Autodesk Fusion 360 part; units mm, degrees
sketch "Outer" plane through (0, 0, 0) normal (0, 1, 0) x (1, 0, 0)
  circle A0 centre (0, 0) radius 12.5
  dimension "d1" = 25
extrude "Outer Extrusion" add sketch "Outer" along normal blind 20
sketch "Inner" plane through (0, 20, 0) normal (0, 1, 0) x (-1, 0, 0)
  circle A0 centre (0, 0) radius 12.5
  circle A1 centre (0, 0) radius 10.5
  dimension "d4" = 21
extrude "Inner Extrusion" cut sketch "Inner" against normal blind 18 contours A1
sketch "Shaft" plane through (0, 2, 0) normal (0, 1, 0) x (-1, 0, 0)
  circle A0 centre (0, 0) radius 10.5
  line L0 (-1.7, 2.5923) -> (-1.7, -2.5923)
  arc A1 (-1.7, -2.5923) -> (-1.7, 2.5923) centre (0, 0) ccw
  arc A2 (-3.7, -3.51) -> (-3.7, 3.51) centre (0, 0) ccw
  line L1 (-3.7, 3.51) -> (-3.7, -3.51)
  dimension "d7" = 6.2
  dimension "d8" = 1.7
  dimension "d9" = 2
extrude "Shaft Extrusion" add sketch "Shaft" along normal blind 12.5 contours A2 L1
equation "d4 = 25 mm - 2 mm - 2 mm"
equation "d5 = -( 20 mm - 2 mm )"
equation "d7 = 5.8 mm + 0.2 mm + 0.2 mm"
equation "d8 = ( 4.5 mm - 3 mm ) + 0.2 mm"
equation "d10 = 20 mm - 2 mm - 5.5 mm"
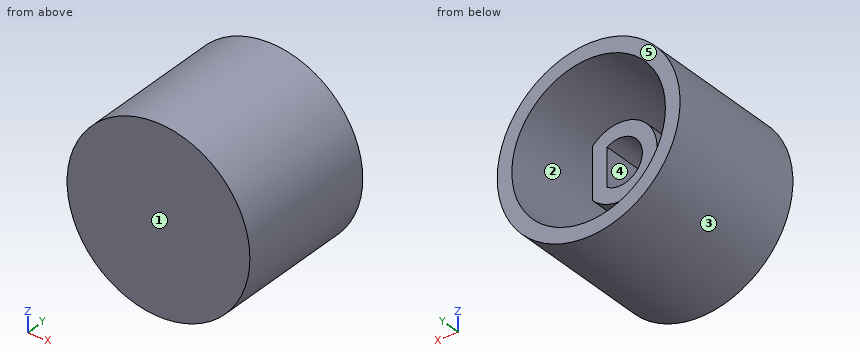
Check sheet for the modelled part. Datum: model origin and axes. Units: mm. Face numbers are marked on the shaded views. A direction names the side the tool comes from. Round coordinates to 2 decimals unless told otherwise and drop trailing zeros. Write each loop counter-clockwise with the first axis right and the second up, starting at its lowest first coordinate (ties: lowest second). Pieces come first, ordered by that corner, then holes. Notation, with made-up numbers: (69.5, -24) - (85.5, -24) arc R35 ccw to (85.5, 15) - close; hole circle Ø11 at (80.25, -25). An arc over 180 degrees is marked (long way). Return JSON: item names as keys, results as strings.
Q1. Cross-section at B-B (z = 0). Record the boundary of the cut face in (x, y).
Returned:
{"outline": "(-12.5, 0) - (12.5, 0) - (12.5, 20) - (10.5, 20) - (10.5, 2) - (3.7, 2) - (3.7, 14.5) - (1.7, 14.5) - (1.7, 2) - (-3.1, 2) - (-3.1, 14.5) - (-5.1, 14.5) - (-5.1, 2) - (-10.5, 2) - (-10.5, 20) - (-12.5, 20) - close"}
Q2. Depth check by flat-ended pin: P1, Ø5.5, axis at x = 0, z = 0, coming from the +Y side; P2, Ø1, axis at x = 5.5, z = -7.5, coming from the -Y side; P3, Ø3, axis at x = 5, y = 6, coming from the +Z side; P4, Ø1, axis at x = 9.5, y = 10.5, coming from the +Z side. Enter the tip coordinate at first touch or a pass-through.
Returned:
{"P1": "stops at y = 14.5", "P2": "stops at y = 0", "P3": "stops at z = 12", "P4": "stops at z = 8.67"}
Q3. Cross-section at C-C (x = 0). Record the boundary of the cut face in (y, z).
Returned:
{"outline": "(0, -12.5) - (20, -12.5) - (20, -10.5) - (2, -10.5) - (2, -5.1) - (14.5, -5.1) - (14.5, -3.1) - (2, -3.1) - (2, 3.1) - (14.5, 3.1) - (14.5, 5.1) - (2, 5.1) - (2, 10.5) - (20, 10.5) - (20, 12.5) - (0, 12.5) - close"}
Q4. Access from +Z, -Z, +X, -X, +Y, -Y to the whole of each face (thin tool, end or side, straight path). Record for the marked faces 1 and 2.
Returned:
{"face 1": "+Z, -Z, +X, -X, -Y", "face 2": "+Y"}
Q5. Draft check along X on the marked faces 3, 4 and 5. Enter one of: released by +X, released by -X, zero draft, split by the parting line, or undercut.
Returned:
{"face 3": "split by the parting line", "face 4": "undercut", "face 5": "zero draft"}
Q6. Scan lines: L1, parallel to Z at x = 0, y = 12.5; L2, parallel to Y at x = -1.25, z = 1; L3, parallel to Z at x = -0.25, y = 16. Record each from-to range of solid material in increasing order. Write a range as from..to.
Returned:
{"L1": "z = -12.5..-10.5, -5.1..-3.1, 3.1..5.1, 10.5..12.5", "L2": "y = 0..2", "L3": "z = -12.5..-10.5, 10.5..12.5"}
Q7. Cross-section at D-D (z = 7.5). Record the boundary of the cut face in (x, y), then the cut area to 3 significant figures.
Returned:
{"outline": "(-10, 0) - (10, 0) - (10, 20) - (7.35, 20) - (7.35, 2) - (-7.35, 2) - (-7.35, 20) - (-10, 20) - close", "area": "135 mm²"}
Q8. Cross-section at A-A (y = 13.75). Record the boundary of the cut face in (x, z), then the cut area to 3 significant figures.
Returned:
{"outline": "circle Ø25 at (0, 0); (3.7, -3.51) - (3.7, 3.51) arc R5.1 ccw (long way) to start; hole circle Ø21 at (0, 0); hole (1.7, -2.59) - (1.7, 2.59) arc R3.1 ccw (long way) to start", "area": "194 mm²"}
